Input: part model. Units: mm. Frame: model coordinates. Round coordinates to 2 decimals unless told otherwise and drop trailing zeros. Loops run counter-clockwise (first coordinate to the right, second up) from the corner with the lowest first, then second, coordinate; pieces in that order, holes last.
(1) Line query: line 1 (Y direction, x = 67.5, z = 8.25); line 2 (X direction, y = -23, z = 29.25). Output: solid intervals per line, ascending.
(2) Cut plane C-C, the plane z = 14.25. Output: boundary loops of the cut face in (x, y), and give its area (3 significant figures).
(3) First-contact query: pin 1 Ø1.5 at (y, z) = (-45, 13.5) entering from -X. Flat tip, straight axial feed; report the tip coordinate or a pass-through.
(4) Cut plane B-B, the plane y = -26. Output: boundary loops of the cut face in (x, z), and give its area (3 significant figures).
(5) Cut plane A-A, the plane x = 7.5. Output: boundary loops of the cut face in (y, z).
(6) Draft query along X for faces 1 (the face through (0, -26, 15)), 2 (the face through (7.04, -22.53, 14.79)), 3 (the face through (37, -52, 15)). Return one class per face: released by +X, released by -X, zero draft, split by the parting line, or undercut.
from build123d import *

# Parameters (mm, degrees)
SKETCH1_W           = 75
SKETCH1_H           = 52
SKETCH1_R           = 3.5
BOSS_EXTRUDE1_DEPTH = 30


with BuildPart() as part:
    # Sketch1 → Boss-Extrude1 (new body)
    with BuildSketch(Plane.XY):
        with Locations((37.5, -26)):
            Rectangle(SKETCH1_W, SKETCH1_H)
        with Locations((7.5, -26)):
            Circle(SKETCH1_R, mode=Mode.SUBTRACT)
        with Locations(Location((67.5, -26, 0), (0, 0, 180))):
            Circle(SKETCH1_R, mode=Mode.SUBTRACT)
    extrude(amount=BOSS_EXTRUDE1_DEPTH)


solid = part.part
Reported:
1. line 1: y = -52 to -29.5, -22.5 to 0
1. line 2: x = 0 to 5.7, 9.3 to 65.7, 69.3 to 75
2. outline: (0, -52) - (75, -52) - (75, 0) - (0, 0) - close; hole circle Ø7 at (7.5, -26); hole circle Ø7 at (67.5, -26)
2. area: 3,820 mm2
3. pin 1: stops at x = 0
4. outline: (0, 0) - (4, 0) - (4, 30) - (0, 30) - close; (11, 0) - (64, 0) - (64, 30) - (11, 30) - close; (71, 0) - (75, 0) - (75, 30) - (71, 30) - close
4. area: 1,830 mm2
5. outline: (-52, 0) - (-29.5, 0) - (-29.5, 30) - (-52, 30) - close; (-22.5, 0) - (0, 0) - (0, 30) - (-22.5, 30) - close
6. face 1: released by -X
6. face 2: undercut
6. face 3: zero draft
